Build history of the part. All positions in model axes, mm. Face numbers are marked on the shaded views. A direction names the side the tool comes from. Round coordinates to 2 decimals unless told otherwise and drop trailing zeros. Order: outer loops, then holes, each group sorted by start corner. A loop starts at its lowest first (then second) coordinate and runs counter-clockwise, first axis right, second up. Notation, with made-up numbers: M 15,40.5 L 70,40.5 A19 cw 70,48.5 Z; hole C -16,85.5 d6. An arc over 180 degrees is marked long. One line per item, written item: value. Start each with the question number.
Item 1: Band-saw the part on D-D, the plane y = 10.5. Write the cut outline in (x, z).
Item 2: Probe L1, parallel to Z at x = 69, y = 4; L2, parallel to Z at x = -65.5, y = 5.75; L3, parallel to Y at x = 3.5, z = 24.5. List the from-to ranges inside material, lowest first.
Item 3: Band-saw the part on C-C, the plane x = 9. Write the cut outline in (y, z), then the cut area to 3 significant figures.
Item 4: Pin check, flat tips, straight feed: pin 1 (3 mm diameter, centred on y = 4, z = 35, fed in from +X); pin 2 (10 mm diameter, centred on x = 38.5, z = -19, fed in from +Y); pin 3 (1.6 mm diameter, centred on x = 69.5, y = 4, fed in from -Z). Stop position of each tip, or through.
Item 5: Two-plate mould, pull along X, no slides. Class the marked faces 1, 2 and 3: +X half, -X half, draft (parallel to the pull), parting line (faces both ways), or undercut.
Item 6: Band-saw the part on B-B, the plane z = 38. Write the cut outline in (x, y), then the cut area to 3 significant figures.
Item 7: Tool access for the marked faces 4 and 5: list every direction of +Z, -Z, +X, -X, +Y, -Y with a clear straight run to the whole face (end or side of a thin tool).
Item 8: Band-saw the part on A-A, the plane z = 54. Write the cut outline in (x, y), then the cut area to 3 significant figures.
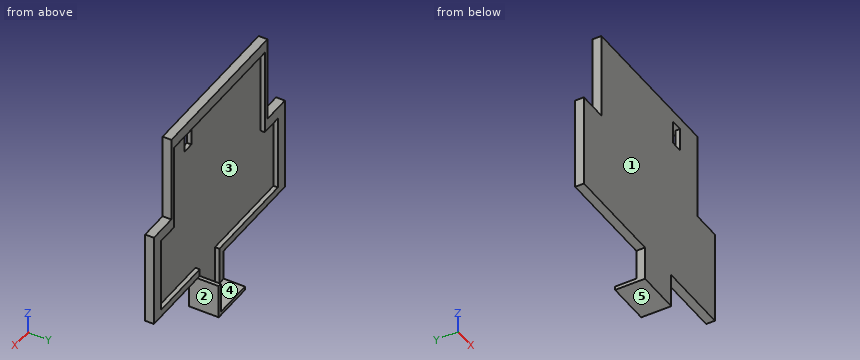
```python
from build123d import *

# Parameters (mm, degrees)
CROQUIS1_W              = 150
CROQUIS1_H              = 148.5
SALIENTE_EXTRUIR1_DEPTH = 6
CROQUIS2_W              = 50
CROQUIS2_H              = 23.5
CROQUIS2_W_2            = 70
CROQUIS2_W_3            = 20
CROQUIS2_H_2            = 60
CORTAR_EXTRUIR2_DEPTH   = 8
CORTAR_EXTRUIR3_DEPTH   = 3
CROQUIS4_W              = 134
CROQUIS4_H              = 3
CROQUIS4_W_2            = 5
CROQUIS4_H_2            = 60
CROQUIS4_W_3            = 22.5
CROQUIS4_H_3            = 5.5
CORTAR_EXTRUIR4_DEPTH   = 3
CROQUIS5_W              = 3
CROQUIS5_H              = 20.5
CROQUIS5_W_2            = 5.5
CORTAR_EXTRUIR5_DEPTH   = 3
SALIENTE_EXTRUIR3_DEPTH = 14.5
CROQUIS8_W              = 6
CROQUIS8_H              = 13
CROQUIS8_W_2            = 13
CROQUIS8_H_2            = 6
CORTAR_EXTRUIR6_DEPTH   = 3
CROQUIS9_W              = 8
CROQUIS9_H              = 16
CORTAR_EXTRUIR7_DEPTH   = 107.978093552
SALIENTE_EXTRUIR4_DEPTH = 1


with BuildPart() as part:
    # Croquis1 → Saliente-Extruir1 (new body)
    with BuildSketch(Plane(origin=(0, 0, 0), x_dir=(1, 0, 0), z_dir=(0, 1, 0))):
        Rectangle(CROQUIS1_W, CROQUIS1_H)
    extrude(amount=SALIENTE_EXTRUIR1_DEPTH)

    # Croquis2 → Cortar-Extruir2 (cut)
    with BuildSketch(Plane(origin=(0, 6, 0), x_dir=(1, 0, 0), z_dir=(0, 1, 0))):
        with Locations((50, 62.5)):
            Rectangle(CROQUIS2_W, CROQUIS2_H)
        with Locations((-40, 62.5)):
            Rectangle(CROQUIS2_W_2, CROQUIS2_H)
        with Locations((-65, -44.25)):
            Rectangle(CROQUIS2_W_3, CROQUIS2_H_2)
        with Locations((65, -44.25)):
            Rectangle(CROQUIS2_W_3, CROQUIS2_H_2)
    extrude(amount=-CORTAR_EXTRUIR2_DEPTH, mode=Mode.SUBTRACT)

    # Croquis3 → Cortar-Extruir3 (cut)
    with BuildSketch(Plane(origin=(0, 6, 0), x_dir=(1, 0, 0), z_dir=(0, 1, 0))):
        Polygon((47, -6.25), (67, -6.25), (67, 42.75), (17, 42.75), (17, 66.25), (3, 66.25), (3, 42.75), (-67, 42.75), (-67, -6.25), (-47, -6.25), (-47, -66.25), (47, -66.25), align=None)
    extrude(amount=-CORTAR_EXTRUIR3_DEPTH, mode=Mode.SUBTRACT)

    # Croquis4 → Cortar-Extruir4 (cut)
    with BuildSketch(Plane(origin=(0, 6, 0), x_dir=(1, 0, 0), z_dir=(0, 1, 0))):
        with Locations((0, 44.25)):
            Rectangle(CROQUIS4_W, CROQUIS4_H)
        with Locations((-49.5, -36.25)):
            Rectangle(CROQUIS4_W_2, CROQUIS4_H_2)
        with Locations((49.5, -36.25)):
            Rectangle(CROQUIS4_W_2, CROQUIS4_H_2)
        with Locations((11.25, 69)):
            Rectangle(CROQUIS4_W_3, CROQUIS4_H_3)
    extrude(amount=-CORTAR_EXTRUIR4_DEPTH, mode=Mode.SUBTRACT)

    # Croquis5 → Cortar-Extruir5 (cut)
    with BuildSketch(Plane(origin=(0, 6, 0), x_dir=(1, 0, 0), z_dir=(0, 1, 0))):
        with Locations((1.5, 56)):
            Rectangle(CROQUIS5_W, CROQUIS5_H)
        with Locations((19.75, 56)):
            Rectangle(CROQUIS5_W_2, CROQUIS5_H)
    extrude(amount=-CORTAR_EXTRUIR5_DEPTH, mode=Mode.SUBTRACT)

    # Croquis7 → Saliente-Extruir3 (add)
    with BuildSketch(Plane(origin=(0, 6, 0), x_dir=(1, 0, 0), z_dir=(0, 1, 0))):
        Polygon((25, 50.75), (25, 74.25), (-5, 74.25), (-5, 71.75), (22.5, 71.75), (22.5, 50.75), align=None)
    extrude(amount=SALIENTE_EXTRUIR3_DEPTH)

    # Croquis8 → Cortar-Extruir6 (cut)
    with BuildSketch(Plane(origin=(0, 6, 0), x_dir=(1, 0, 0), z_dir=(0, 1, 0))):
        with Locations((-71, 18.25)):
            Rectangle(CROQUIS8_W, CROQUIS8_H)
        with Locations((71, 18.25)):
            Rectangle(CROQUIS8_W, CROQUIS8_H)
        with Locations((0, -70.25)):
            Rectangle(CROQUIS8_W_2, CROQUIS8_H_2)
    extrude(amount=-CORTAR_EXTRUIR6_DEPTH, mode=Mode.SUBTRACT)

    # Croquis9 → Cortar-Extruir7 (cut, through all)
    with BuildSketch(Plane(origin=(0, 3, 0), x_dir=(1, 0, 0), z_dir=(0, 1, 0))):
        with Locations((31, -58.25)):
            Rectangle(CROQUIS9_W, CROQUIS9_H)
    extrude(amount=-CORTAR_EXTRUIR7_DEPTH, mode=Mode.SUBTRACT)

    # Croquis10 → Saliente-Extruir4 (add)
    with BuildSketch(Plane(origin=(0, 6, 0), x_dir=(1, 0, 0), z_dir=(0, 1, 0))):
        Polygon((25, 50.75), (22.5, 50.75), (22.5, 45.75), (67, 45.75), (67, -6.25), (52, -6.25), (52, -66.25), (-52, -66.25), (-52, -6.25), (-67, -6.25), (-67, 45.75), (0, 45.75), (0, 71.75), (-5, 71.75), (-5, 50.75), (-75, 50.75), (-75, -14.25), (-55, -14.25), (-55, -74.25), (55, -74.25), (55, -14.25), (75, -14.25), (75, 50.75), align=None)
    extrude(amount=-SALIENTE_EXTRUIR4_DEPTH)


solid = part.part
```
Output:
1. outline: M -5,-74.25 L 25,-74.25 L 25,-50.75 L 22.5,-50.75 L 22.5,-71.75 L -5,-71.75 Z
2. L1: z = -50.75 to -24.75, -11.75 to 14.25
2. L2: z = -50.75 to -45.75, 6.25 to 14.25
2. L3: y = 0 to 3
3. outline: M 0,-74.25 L 20.5,-74.25 L 20.5,-71.75 L 3,-71.75 L 3,66.25 L 6,66.25 L 6,74.25 L 0,74.25 Z
3. area: 513 mm²
4. pin 1: stops at x = 55
4. pin 2: stops at y = 3
4. pin 3: stops at z = -50.75
5. face 1: draft
5. face 2: +X half
5. face 3: undercut
6. outline: M -55,0 L 55,0 L 55,6 L 52,6 L 52,3 L -52,3 L -52,6 L -55,6 Z
6. area: 348 mm²
7. face 4: +Y
7. face 5: -Z, +X, -X, +Y, -Y
8. outline: M -55,0 L 27,0 L 27,3 L -52,3 L -52,6 L -55,6 Z; M 35,0 L 55,0 L 55,6 L 52,6 L 52,3 L 35,3 Z
8. area: 324 mm²
